Geometry check sheet. Reference: the model listing, model coordinates, mm. A direction names the side the tool comes from. Round coordinates to 2 decimals unless told otherwise and drop trailing zeros. Order: outer loops, then holes, each group sorted by start corner. A loop starts at its lowest first (then second) coordinate and runs counter-clockwise, first axis right, second up.
```python
from build123d import *

# Parameters (mm, degrees)
F1_DEPTH = 19.05
F2_DEPTH = 25.4
F3_W     = 19.790456
F3_H     = 6.35
F4_DEPTH = 6.35
F5_R     = 3.175
F6_DEPTH = 19.05


with BuildPart() as f1:
    # F0 (on Front) → F1 (new body)
    with BuildSketch(Plane.XZ):
        Polygon((0, 14.418764), (0, 0), (6.7853, 0), (6.7853, 8.387386), (22.99463, 8.387386), (22.99463, 14.418764), align=None)
    extrude(amount=F1_DEPTH)

    # F0 (on Front) → F2 (join)
    with BuildSketch(Plane.XZ):
        Polygon((22.99463, 24.973674), (22.99463, 14.418764), (22.99463, 8.387386), (42.785086, 8.198905), (42.785086, 24.973674), align=None)
    extrude(amount=F2_DEPTH)

    # F3 (on face) → F4 (join)
    with BuildSketch(Plane.XY.offset(24.973674)):
        with Locations((32.889858, -3.175)):
            Rectangle(F3_W, F3_H)
    extrude(amount=F4_DEPTH)

    # F5 (on face) → F6 (cut, symmetric)
    with BuildSketch(Plane(origin=(0.081958, 0, 8.605602), x_dir=(0.999955, 0, -0.009523), z_dir=(-0.009523, 0, -0.999955))):
        with Locations((16.563711, 9.525)):
            Circle(F5_R)
        with Locations((32.438711, 9.525)):
            Circle(F5_R)
    extrude(amount=F6_DEPTH, both=True, mode=Mode.SUBTRACT)


solid = f1.part
```
(1) Sectioned sample at A-A, the plane y = -13.25. Record the cut outline in (x, z), and give its area (3 significant figures).
Returned:
outline: (0, 0) - (6.79, 0) - (6.79, 8.39) - (22.99, 8.39) - (42.79, 8.2) - (42.79, 24.97) - (22.99, 24.97) - (22.99, 14.42) - (0, 14.42) - close
area: 526 mm2
(2) Sectioned sample at C-C, the plane z = 6. Record the cut outline in (x, y).
Returned:
outline: (0, -19.05) - (6.79, -19.05) - (6.79, 0) - (0, 0) - close
(3) Depth check by flat-ended pin: P1, Ø5.5, axis at x = 7, y = -13, coming from the +Z side; P2, Ø9.5, axis at x = 37.5, y = -15.5, coming from the +Z side; P3, Ø4.5, axis at x = 7, z = 10.5, coming from the -Y side; P4, Ø6, axis at x = 15.5, z = 18, coming from the +Y side. Enter the tip coordinate at first touch or a pass-through.
Returned:
P1: stops at z = 14.42
P2: stops at z = 24.97
P3: stops at y = -19.05
P4: passes through
(4) Draft check along X on faces 1 (the cylindrical face through (35.626, -10.479, 16.505)), 2 (the flat face through (42.785, -13, 17)), 3 (the flat face through (3, -9, 0)). Enter one of: released by +X, released by -X, zero draft, split by the parting line, or undercut.
Returned:
face 1: undercut
face 2: released by +X
face 3: zero draft
(5) Material ranges on line 1 (Z direction, x = 22.5, y = -11.5); line 2 (Y direction, x = 24.5, z = 27); line 3 (X direction, y = -13, z = 16), recorded low to high.
Returned:
line 1: z = 8.39 to 14.42
line 2: y = -6.35 to 0
line 3: x = 22.99 to 42.79
(6) Sectioned sample at B-B, the plane x = 28.5. Record the cut outline in (y, z).
Returned:
outline: (-25.4, 8.33) - (0, 8.33) - (0, 31.32) - (-6.35, 31.32) - (-6.35, 24.97) - (-25.4, 24.97) - close
(7) Sectioned sample at D-D, the plane y = -2.5. Record the cut outline in (x, z), and give its area (3 significant figures).
Returned:
outline: (0, 0) - (6.79, 0) - (6.79, 8.39) - (22.99, 8.39) - (42.79, 8.2) - (42.79, 31.32) - (22.99, 31.32) - (22.99, 14.42) - (0, 14.42) - close
area: 651 mm2
(8) Set-up check for faces 4 (the flat face through (13, -9, 8.387)), 5 (the flat face through (9, -19.05, 9)), 6 (the cylindrical face through (14.33, -11.67, 11.38)), 7 (the flat face through (33, -6.35, 28)): record each of +Z, -Z, +X, -X, +Y, -Y from which the full face is reachable in a straight line by a thin tool's end or side.
Returned:
face 4: -Z, +Y, -Y
face 5: +Z, -Z, -X, -Y
face 6: none
face 7: +Z, +X, -X, -Y
